Autodesk Inventor part; units mm, degrees
ref_plane "YZ Plane" through (0, 0, 0) normal (1, 0, 0) x (0, 1, 0)
ref_plane "XZ Plane" through (0, 0, 0) normal (0, 1, 0) x (-1, 0, 0)
ref_plane "XY Plane" through (0, 0, 0) normal (0, 0, 1) x (1, 0, 0)
sketch "Sketch1" plane through (0, 0, 0) normal (0, 0, 1) x (1, 0, 0)
  line L0 (0, 0) -> (6, 0)
  line L1 (6, 0) -> (6, 6)
  line L2 (6, 6) -> (0, 6)
  line L3 (0, 6) -> (0, 0)
  dimension "d0" = 6
  dimension "d1" = 6
extrude "Extrusion1" add sketch "Sketch1" along normal blind 1
sketch "Sketch2" plane through (0, 0, 1) normal (0, 0, 1) x (1, 0, 0)
  circle A0 centre (3, 3) radius 3
  line L0 (0, 6) -> (0, 0)
  line L1 (0, 0) -> (6, 0)
  dimension "d4" = 6
  dimension "d5" = 3
  dimension "d6" = 3
extrude "Extrusion2" add sketch "Sketch2" along normal blind 2.5 contours A0
properties part number "Servo_bit"
The listing builds one solid part. Answer for the finished solid, in the listing's coordinates (mm). A direction names the side the tool comes from. Give positions to 0.01 mm unless a question says otherwise; leave off trailing zeros. Order: outer loops, then holes, each group sorted by start corner. A loop starts at its lowest first (then second) coordinate and runs counter-clockwise, first axis right, second up. Notation, with made-up numbers: (9, -11.75) - (17, -11.75) arc R11 cw to (17, 9.25) - close; hole circle Ø7 at (-37, -24.5). An arc over 180 degrees is marked (long way). One line per item, written item: value. Start each with the question number.
1) A cutting plane is placed at B-B on x = 1.8. Give the vertices of the cut face in (y, z).
2) A tool of negligible diameter and unlimited length cuts with its end or side. For faces 1 (the face through (0.6, 5.3, 1)), 2 (the face through (0.6, 0.7, 1)), 3 (the face through (5.3, 5.4, 1)), 4 (the face through (0.6, 4.8, 2.2)), from which of +Z, -Z, +X, -X, +Y, -Y can it reach the whole face along a straight path? Write none if from no direction.
3) A cutting plane is placed at A-A on y = 5.05. Give the vertices of the cut face in (x, z).
4) Find the intervals of material crossed by L1, parallel to Z at x = 4.4, y = 5.75; L2, parallel to Y at x = 2.5, z = 1.5; L3, parallel to Y at x = 1.65, z = 2.6, in increasing order.
5) A cutting plane is placed at C-C on z = 2.7. Give the vertices of the cut face in (x, y).
Answer sheet:
1. outline: (0, 0) - (6, 0) - (6, 1) - (5.75, 1) - (5.75, 3.5) - (0.25, 3.5) - (0.25, 1) - (0, 1) - close
2. face 1: +Z, -X, +Y
2. face 2: +Z, -X, -Y
2. face 3: +Z, +X, +Y
2. face 4: +Z
3. outline: (0, 0) - (6, 0) - (6, 1) - (5.19, 1) - (5.19, 3.5) - (0.81, 3.5) - (0.81, 1) - (0, 1) - close
4. L1: z = 0 to 1
4. L2: y = 0.04 to 5.96
4. L3: y = 0.32 to 5.68
5. outline: circle Ø6 at (3, 3)
